The model under review builds one solid part; all positions refer to its coordinate system, in mm. Face numbers are marked on the shaded views. Coordinates: 2 decimals unless noted, no trailing zeros. Loops run counter-clockwise (first coordinate to the right, second up) from the corner with the lowest first, then second, coordinate; pieces in that order, holes last. Notation, with made-up numbers: M 65,88.25 L 119,88.25 A15 cw 119,96.25 Z; hole C 15.25,-14.75 d6. An arc over 180 degrees is marked long. Use CSV: the item, a comma, the result in double quotes. Start each with the question number.
1. Add section C-C, the plane z = 0. Write out the cut boundary in (x, y), then the cut area to 3 significant figures.
2. Clearance check with flat-ended pins moving along their axes: P1, Ø1, axis at x = -8.5, z = 2.5, coming from the +Y side; P2, Ø3, axis at x = 0, z = 0, coming from the +Y side. State where each tip first meets the part, or that it passes through.
3. For L1, parallel to Z at x = 0, y = 0.25; L2, parallel to Y at x = -2, z = 13; L3, parallel to X at y = 1.5, z = -6, list the stretches that pass through material, from the lowest coordinate up.
4. Draft analysis for pull direction X (two halves, no side actions). For the marked faces 1 and 2, state which applies: +X half, -X half, draft (parallel to the pull), parting line (faces both ways), or undercut.
5. Add section D-D, the plane y = 0.55. Write out the cut boundary in (x, z), then the cut area to 3 significant figures.
6. Add section B-B, the plane y = 2.6. Write out the cut boundary in (x, z).
7. Add section A-A, the plane x = 0. Write out the cut boundary in (y, z), then the cut area to 3 significant figures.
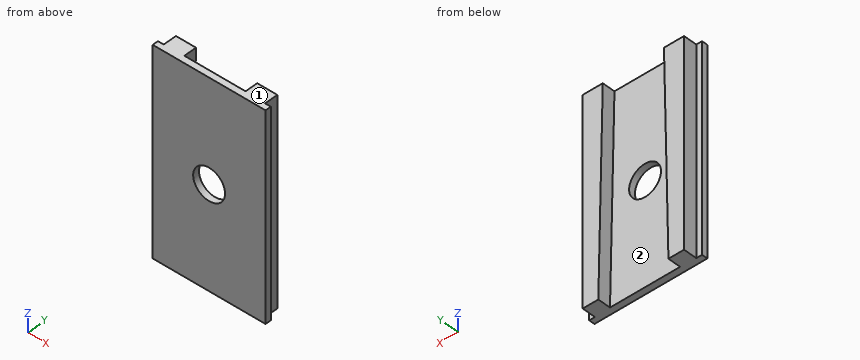
Autodesk Inventor part; units mm, degrees
ref_plane "YZ Plane" through (0, 0, 0) normal (1, 0, 0) x (0, 1, 0)
ref_plane "XZ Plane" through (0, 0, 0) normal (0, 1, 0) x (-1, 0, 0)
ref_plane "XY Plane" through (0, 0, 0) normal (0, 0, 1) x (1, 0, 0)
sketch "Sketch1" plane through (0, 0, 0) normal (0, 1, 0) x (-1, 0, 0)
  line L0 (7.95, 15.98) -> (-7.95, 15.98)
  line L1 (-7.95, 15.98) -> (-7.95, -15.98)
  line L2 (-7.95, -15.98) -> (7.95, -15.98)
  line L3 (7.95, -15.98) -> (7.95, 15.98)
  line L4 (7.95, 15.98) -> (-7.95, -15.98) construction
  line L5 (-7.95, 15.98) -> (7.95, -15.98) construction
  point P0 (0, 0)
  dimension "d0" = 31.96
  dimension "d1" = 15.9
extrude "adapter-arm" add sketch "Sketch1" along normal blind 3
sketch "fanslot" plane through (0, 3, 0) normal (0, 1, 0) x (1, 0, 0)
  line L0 (-4.8, -15.98) -> (4.8, -15.98)
  line L1 (4.8, -15.98) -> (5.5, 15.98)
  line L2 (5.5, 15.98) -> (-5.5, 15.98)
  line L3 (-5.5, 15.98) -> (-4.8, -15.98)
  line L4 (0, 16.157) -> (0, -15.9695) construction
  line L5 (-7.95, -15.98) -> (7.95, -15.98) construction
  line L6 (7.95, 15.98) -> (-7.95, 15.98) construction
  point P0 (0, 0)
  point P1 (0, -15.98)
  point P2 (0, 15.98)
  point P3 (-5.98, -15.98)
  point P4 (5.98, -15.98)
  point P5 (5.98, 15.98)
  point P6 (-5.98, 15.98)
  dimension "d21" = 11
  dimension "d22" = 9.6
extrude "Extrusion3" cut sketch "fanslot" against normal blind 2
sketch "Sketch5" plane through (0, 0, 0) normal (0, -1, 0) x (1, 0, 0)
  circle A0 centre (0, 0) radius 2.5
  dimension "d25" = 5
extrude "Extrusion4" cut sketch "Sketch5" against normal up to next
sketch "Sketch6" plane through (-7.95, 0, 15.98) normal (0, 0, 1) x (1, 0, 0)
  line L0 (0, 0) -> (-0.9, 0)
  line L1 (-0.9, 0) -> (-0.9, 0.9)
  line L2 (-0.9, 0.9) -> (0, 0.9)
  line L3 (0, 0.9) -> (0, 0)
  line L4 (15.9, 0) -> (16.8, 0)
  line L5 (16.8, 0) -> (16.8, 0.9)
  line L6 (16.8, 0.9) -> (15.9, 0.9)
  line L7 (15.9, 0.9) -> (15.9, 0)
  point P0 (7.95, 0)
  dimension "d28" = 0.9
  dimension "d29" = 0.9
  dimension "d30" = 0.9
  dimension "d31" = 0.9
extrude "Extrusion5" add sketch "Sketch6" against normal up to surface (31.96 mm away)
equation "\"d2\" = armthick"
equation "\"d21\" = fanhb"
equation "\"d22\" = fanhs"
equation "\"d23\" = armslotd"
equation "\"printer3dtolerance\" = 0.1"
equation "\"wallw\" = 42"
equation "\"wallh\" = 44"
equation "\"cornerrad\" = 2"
equation "\"baseextra\" = 2"
equation "\"wall1_thick\" = 8"
equation "\"wall2_thick\" = 6.4"
equation "\"wall3_thick\" = 4"
equation "\"wall1slot\" = 8.1"
equation "\"wall2slot\" = 6.5"
equation "\"wall3slot\" = 4.1"
equation "\"gap2\" = 28"
equation "\"baseh\" = 79"
equation "\"basew\" = 44"
equation "\"base_thick\" = 6"
equation "\"base_slots_depth\" = 4"
equation "\"servobigcircledia\" = 11.6"
equation "\"servosmallcircledia\" = 5.9"
equation "\"servo9gw\" = 22.8"
equation "\"servomounth\" = 4"
equation "\"servomountsquare\" = 4"
equation "\"servopolygonr\" = 6.1"
equation "\"servopolygonl\" = 5.9"
equation "\"distancefrombottom\" = 34"
equation "\"distancefromleft\" = 22"
equation "\"wall3slotd\" = 2"
equation "\"wall3slotw\" = 36"
equation "\"adapterh\" = 16"
equation "\"adapterw\" = 32"
equation "\"armw\" = 34"
equation "\"armslotd\" = 2"
equation "\"armthick\" = 3"
equation "\"fanhb\" = 11"
equation "\"fanhs\" = 9.6"
equation "\"adapterwallthick\" = 6"
equation "\"adapterwallslotd\" = 2"
equation "\"hornscrewheadd\" = 3"
equation "\"hornscrewholed\" = 2"
equation "\"hornthick\" = 1.5"
equation "\"armhornthick\" = 3"
properties part number "adapter-slot"
Computed:
1,outline,"M -8.85,0 L -2.5,0 L -2.5,1 L -5.15,1 L -5.15,3 L -7.95,3 L -7.95,0.9 L -8.85,0.9 Z; M 2.5,0 L 8.85,0 L 8.85,0.9 L 7.95,0.9 L 7.95,3 L 5.15,3 L 5.15,1 L 2.5,1 Z"
1,area,"23.7 mm^2"
2,P1,"stops at y = 0.9"
2,P2,"passes through"
3,L1,"z = -15.98 to -2.5, 2.5 to 15.98"
3,L2,"y = 0 to 1"
3,L3,"x = -7.95 to -5.28, 5.28 to 7.95"
4,face 1,"draft"
4,face 2,"undercut"
5,outline,"M -8.85,-15.98 L 8.85,-15.98 L 8.85,15.98 L -8.85,15.98 Z; hole C 0,0 d5"
5,area,"546 mm^2"
6,outline,"M -7.95,-15.98 L -5.5,-15.98 L -4.8,15.98 L -7.95,15.98 Z; M 4.8,15.98 L 5.5,-15.98 L 7.95,-15.98 L 7.95,15.98 Z"
7,outline,"M 0,-15.98 L 1,-15.98 L 1,-2.5 L 0,-2.5 Z; M 0,2.5 L 1,2.5 L 1,15.98 L 0,15.98 Z"
7,area,"27.0 mm^2"
